```python
from build123d import *

# Parameters (mm, degrees)
F0_W      = 110
F0_H      = 105
F1_DEPTH  = 5
F2_W      = 110
F2_H      = 5
F3_DEPTH  = 100
F5_DEPTH  = 5
F8_DEPTH  = 5.001
F10_DEPTH = 105.001
F11_SIZE  = 5


with BuildPart() as f1:
    # F0 (on Top) → F1 (new body)
    with BuildSketch(Plane.XY):
        Rectangle(F0_W, F0_H)
    extrude(amount=F1_DEPTH)

    # F2 (on face) → F3 (join)
    with BuildSketch(Plane.XY.offset(5)):
        with Locations((0, 50)):
            Rectangle(F2_W, F2_H)
    extrude(amount=F3_DEPTH)

    # F4 (on face) → F5 (join)
    with BuildSketch(Plane(origin=(-55, 0, 0), x_dir=(0, -1, 0), z_dir=(-1, 0, 0))):
        with BuildLine():
            ThreePointArc((52.5, 5), (-18.2106781187, 34.2893218813), (-47.5, 105))
            Line((-47.5, 105), (-47.5, 72.9843788128))
            ThreePointArc((-47.5, 72.9843788128), (-21.7462120246, 30.7537879754), (20.4843788128, 5))
            Line((20.4843788128, 5), (52.5, 5))
        make_face()
    extrude(amount=-F5_DEPTH)

    # F6: F1 across plane


with BuildPart() as f1_1:
    add(f1.part)
    add(f1.part.mirror(Plane.YZ))

    # F7 (on face) → F8 (cut, through all)
    with BuildSketch(Plane.XY.offset(5)):
        with BuildLine():
            Line((44.5, -52.5), (44.5, 0))
            ThreePointArc((44.5, 0), (0, 44.5), (-44.5, 0))
            Line((-44.5, 0), (-44.5, -52.5))
            Line((-44.5, -52.5), (44.5, -52.5))
        make_face()
    extrude(amount=-F8_DEPTH, mode=Mode.SUBTRACT)

    # F9 (on face) → F10 (cut, through all)
    with BuildSketch(Plane(origin=(0, 52.5, 0), x_dir=(-1, 0, 0), z_dir=(0, 1, 0))):
        with BuildLine():
            Line((-44.5, 105), (-44.5, 52.5))
            ThreePointArc((-44.5, 52.5), (0, 8), (44.5, 52.5))
            Line((44.5, 52.5), (44.5, 105))
            Line((44.5, 105), (-44.5, 105))
        make_face()
    extrude(amount=-F10_DEPTH, mode=Mode.SUBTRACT)

    # F11
    f11_edges = [f1_1.edges().sort_by_distance(p)[0] for p in [
        (44.5, 50, 105),
        (-44.5, 50, 105),
        (44.5, -52.5, 2.5),
        (-44.5, -52.5, 2.5),
    ]]
    chamfer(f11_edges, length=F11_SIZE)


solid = f1_1.part
```
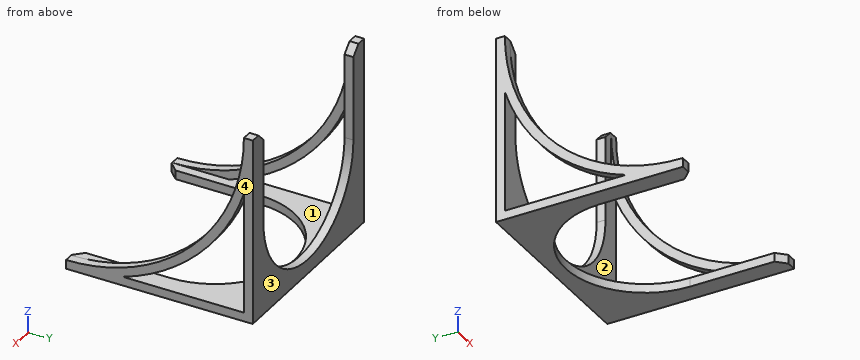
Here's how the part is built. I have some questions about the finished solid (model axes, mm). Face numbers are marked on the shaded views. Round coordinates to 2 decimals unless told otherwise and drop trailing zeros. Write each loop counter-clockwise with the first axis right and the second up, starting at its lowest first coordinate (ties: lowest second). Pieces come first, ordered by that corner, then holes. Notation, with made-up numbers: M 38.5,46 L 80.5,46 A27 ccw 80.5,83 Z; hole C 20.5,2.25 d7. An arc over 180 degrees is marked long. Answer as CSV lines item,"result". Start each with the question number.
1. I need wall thicknesses on probe 1 along X at (y, z) = (-1, 16.5); probe 2 along X at (y, z) = (48.5, 71); probe 3 along Z at (x, y) = (-47, -38). Which ranges of each line are inside material? Lowest first, please.
2. Suppose I cut it at C-C on z = 18. Write out the boundary of the cut face in (x, y), then the cut area to 3 significant figures.
3. Thinking about a two-plate mould opening in Y: for the marked faces 1, 2, 3 and 4, which applies, released by +Y, released by -Y, zero draft, split by the parting line, or undercut?
4. Suppose I cut it at B-B on y = -36. Write out the boundary of the cut face in (x, z), then the cut area to 3 significant figures.
5. I'm going to push a flat-ended pin straight in: pin 1 Ø5 at (x, y) = (-39, 34.5) entering from -Z. Where does the tip first touch, or does it pass through?
6. Suppose I cut it at A-A on z = 97.5. Write out the boundary of the cut face in (x, y).
7. Suppose I cut it at D-D on x = 0. Write out the boundary of the cut face in (y, z), then the cut area to 3 significant figures.
Check result:
1,probe 1,"x = -55 to -50, 50 to 55"
1,probe 2,"x = -55 to -44.5, 44.5 to 55"
1,probe 3,"z = 0 to 5"
2,outline,"M -55,-3.19 L -50,-3.19 L -50,6.29 L -55,6.29 Z; M -55,47.5 L -28.11,47.5 L -28.11,52.5 L -55,52.5 Z; M 28.11,47.5 L 55,47.5 L 55,52.5 L 28.11,52.5 Z; M 50,-3.19 L 55,-3.19 L 55,6.29 L 50,6.29 Z"
2,area,"364 mm2"
3,face 1,"undercut"
3,face 2,"undercut"
3,face 3,"released by +Y"
3,face 4,"zero draft"
4,outline,"M -55,0 L -44.5,0 L -44.5,5 L -50,5 L -50,6.37 L -55,6.37 Z; M 44.5,0 L 55,0 L 55,6.37 L 50,6.37 L 50,5 L 44.5,5 Z"
4,area,"119 mm2"
5,pin 1,"stops at z = 0"
6,outline,"M -55,47.22 L -50,47.22 L -50,47.5 L -44.5,47.5 L -44.5,52.5 L -55,52.5 Z; M 44.5,47.5 L 50,47.5 L 50,47.22 L 55,47.22 L 55,52.5 L 44.5,52.5 Z"
7,outline,"M 44.5,0 L 52.5,0 L 52.5,8 L 47.5,8 L 47.5,5 L 44.5,5 Z"
7,area,"55.0 mm2"
